```python
from build123d import *

# Parameters (mm, degrees)
SKETCH1_W           = 106.1085
SKETCH1_H           = 34.036
BOSS_EXTRUDE1_DEPTH = 13.5001
FILLET1_R           = 2.54
SKETCH4_W           = 8.4963
SKETCH4_H           = 11.938
BOSS_EXTRUDE2_DEPTH = 8.128
FILLET2_R           = 2.54


with BuildPart() as part:
    # Sketch1 → Boss-Extrude1 (new, symmetric)
    with BuildSketch(Plane(origin=(0, 0, 0), x_dir=(1, 0, 0), z_dir=(0, 1, 0))):
        Rectangle(SKETCH1_W, SKETCH1_H)
    extrude(amount=BOSS_EXTRUDE1_DEPTH, both=True)

    # Fillet1
    fillet1_edges = [part.edges().sort_by_distance(p)[0] for p in [
        (-53.05425, 13.5001, 0),
        (0, 13.5001, 17.018),
        (53.05425, 13.5001, 0),
        (0, -13.5001, 17.018),
        (-53.05425, -13.5001, 0),
        (0, -13.5001, -17.018),
        (53.05425, -13.5001, 0),
        (0, 13.5001, -17.018),
    ]]
    fillet(fillet1_edges, radius=FILLET1_R)

    # Sketch4 → Boss-Extrude2 (add)
    with BuildSketch(Plane(origin=(0, 0, -17.018), x_dir=(-1, 0, 0), z_dir=(0, 0, -1))):
        with Locations((50.5079, 0)):
            Rectangle(SKETCH4_W, SKETCH4_H)
    extrude(amount=BOSS_EXTRUDE2_DEPTH)

    # Fillet2
    fillet2_edges = [part.edges().sort_by_distance(p)[0] for p in [
        (-49.657, 5.969, -17.018),
        (-46.25975, 0, -17.018),
        (-49.657, -5.969, -17.018),
    ]]
    fillet(fillet2_edges, radius=FILLET2_R)


solid = part.part
```
The model under review builds one solid part; all positions refer to its coordinate system, in mm. A direction names the side the tool comes from. Round coordinates to 2 decimals unless told otherwise and drop trailing zeros. Order: outer loops, then holes, each group sorted by start corner. A loop starts at its lowest first (then second) coordinate and runs counter-clockwise, first axis right, second up. Notation, with made-up numbers: (-40, 36) - (-4, 36) arc R21 cw to (-4, 71) - close; hole circle Ø4 at (76, -6.5). An arc over 180 degrees is marked (long way). Answer in a Markdown table with one row per item.
(1) Machinability: for faces 1 (the face through (-46.26, 0, -22)), 2 (the face through (-49.49, 6.693, -17.782)), which of the approach directions +Z, -Z, +X, -X, +Y, -Y give a long, thin tool a straight path to every point of the face, cutting with its end or side? Answer none if there is none.
Result set:
| item | result |
|---|---|
| face 1 | -Z, +X, +Y, -Y |
| face 2 | -Z, +X, -X, +Y |
(2) For line 1 (X direction, y = -1.75, z = -21); line 2 (Z direction, x = 0, y = 10.5); line 3 (X direction, y = -7.75, z = 1), list the stretches that pass through material, from the lowest coordinate up. Write a range as from..to.
Result set:
| item | result |
|---|---|
| line 1 | x = -54.76..-46.26 |
| line 2 | z = -17.02..17.02 |
| line 3 | x = -53.05..53.05 |
(3) Take a section at A-A on x = -5. Write out the cut boundary in (y, z), plus the area to 3 significant figures.
Result set:
| item | result |
|---|---|
| outline | (-13.5, -14.48) arc R2.54 ccw to (-10.96, -17.02) - (10.96, -17.02) arc R2.54 ccw to (13.5, -14.48) - (13.5, 14.48) arc R2.54 ccw to (10.96, 17.02) - (-10.96, 17.02) arc R2.54 ccw to (-13.5, 14.48) - close |
| area | 913 mm2 |
(4) Clearance check with flat-ended pins moving along their axes: P1, Ø4, axis at x = 9.5, y = 1, coming from the -Z side; P2, Ø6, axis at y = 0, z = -23.5, coming from the +X side; P3, Ø2.5, axis at x = -49, z = -22.5, coming from the +Y side. State where each tip first meets the part, or that it passes through.
Result set:
| item | result |
|---|---|
| P1 | stops at z = -17.02 |
| P2 | stops at x = -46.26 |
| P3 | stops at y = 5.97 |
(5) Take a section at B-B on z = 9.5. Write out the cut boundary in (x, y), plus the area to 3 significant figures.
Result set:
| item | result |
|---|---|
| outline | (-53.05, -10.96) arc R2.54 ccw to (-50.51, -13.5) - (50.51, -13.5) arc R2.54 ccw to (53.05, -10.96) - (53.05, 10.96) arc R2.54 ccw to (50.51, 13.5) - (-50.51, 13.5) arc R2.54 ccw to (-53.05, 10.96) - close |
| area | 2,860 mm2 |
(6) Take a section at C-C on y = -2.5. Write out the cut boundary in (x, z).
Result set:
| item | result |
|---|---|
| outline | (-54.76, -25.15) - (-46.26, -25.15) - (-46.26, -19.56) arc R2.54 cw to (-43.72, -17.02) - (53.05, -17.02) - (53.05, 17.02) - (-53.05, 17.02) - (-53.05, -17.02) - (-54.76, -17.02) - close |
(7) Take a section at D-D on y = -9.5. Write out the cut boundary in (x, z).
Result set:
| item | result |
|---|---|
| outline | (-53.05, -17.02) - (53.05, -17.02) - (53.05, 17.02) - (-53.05, 17.02) - close |
